CAD build for the part. Positions are in the model's coordinates, mm. A direction names the side the tool comes from. Give positions to 0.01 mm unless a question says otherwise; leave off trailing zeros. Order: outer loops, then holes, each group sorted by start corner. A loop starts at its lowest first (then second) coordinate and runs counter-clockwise, first axis right, second up. Notation, with made-up numbers: M 83.5,58 L 104.5,58 A29 cw 104.5,90 Z; hole C -8,-11.75 d4. An arc over 180 degrees is marked long. Put each result on its own line as item: value. Start each with the question number.
1) Cut at B-B (z = -1.5). Give the number of separate pieces and of enclosed holes in the cut face, and give its area (3 significant figures).
2) Pin check, flat tips, straight feed: pin 1 (5.5 mm diameter, centred on y = -20.5, z = -19, fed in from +X); pin 2 (9.5 mm diameter, centred on x = -62, y = -1.5, fed in from +Z); pin 3 (5.5 mm diameter, centred on x = 10.77, y = -29.6, fed in from -Z); pin 4 (4 mm diameter, centred on x = -26.57, y = 26.92, fed in from +Z). Stop position of each tip, or through.
3) Two-plate mould, pull along X, no slides. Class faces 1 (the face through (56.65, 5.06, -27.46)), 2 (the face through (-1, 1, 0)), 3 (the face through (50, 1, -15)): released by +X, released by -X, zero draft, split by the parting line, or undercut.
4) Drill centre lines: line 1 (X direction, y = -24.5, z = -27.5); line 2 (X direction, y = -0.5, z = -17.5); line 3 (Z direction, x = 61, y = 28.5). Where is each one in solid material? Low to high. Write a range as [from, to].
5) Cut at C-C (x = -40). Write the cut outline in (y, z), and give its area (3 significant figures).
6) Tool access for faces 4 (the face through (-56.65, 5.06, -27.46)), 5 (the face through (48.275, 0.672, -1.636)): list every direction of +Z, -Z, +X, -X, +Y, -Y with a clear straight run to the whole face (end or side of a thin tool).
7) Cut at A-A (z = -11). Write the cut outline in (x, y).
```python
from build123d import *

# Parameters (mm, degrees)
ESBO_O1_W                      = 100
ESBO_O1_H                      = 96
FLANGE_BASE1_DEPTH             = 5
ARESTA_FLANGE1_STRIP_W         = 21.4732
ARESTA_FLANGE1_STRIP_H         = 5
ARESTA_FLANGE1_STRIP_CUT_DEPTH = 96
ARESTA_FLANGE1_DEPTH           = 96
ARESTA_FLANGE2_STRIP_W         = 21.4732
ARESTA_FLANGE2_STRIP_H         = 5
ARESTA_FLANGE2_STRIP_CUT_DEPTH = 96
ARESTA_FLANGE2_DEPTH           = 96
ARESTA_FLANGE3_STRIP_W         = 21.4732
ARESTA_FLANGE3_STRIP_H         = 5
ARESTA_FLANGE3_STRIP_CUT_DEPTH = 96
ARESTA_FLANGE3_DEPTH           = 96
ARESTA_FLANGE4_STRIP_W         = 21.4732
ARESTA_FLANGE4_STRIP_H         = 5
ARESTA_FLANGE4_STRIP_CUT_DEPTH = 96
ARESTA_FLANGE4_DEPTH           = 96
FURO_DE_DI_METRO_4_2_4_2_1_D   = 4.2
PADR_OCIRCULAR1_COUNT          = 8
FURO_DE_DI_METRO_4_2_4_2_2_D   = 4.2
PADR_OCIRCULAR2_COUNT          = 8
FURO_DE_DI_METRO_4_2_4_2_3_D   = 4.2
PADR_OCIRCULAR3_COUNT          = 8
CORTE_EXTRUS_O1_REACH          = 90.482
PADR_O_LINEAR2_COUNT           = 6
PADR_O_LINEAR2_PITCH           = 15
ESPELHAR2_COPY_1_REACH         = 90.482
ESPELHAR2_COPY_2_REACH         = 90.482
ESPELHAR2_COPY_3_REACH         = 90.482
ESPELHAR2_COPY_4_REACH         = 90.482
ESPELHAR2_COPY_5_REACH         = 90.482


# Sheet-metal steps are written as plain solids
with BuildPart() as part:
    # Esboço1 → Flange-base1 (new body)
    with BuildSketch(Plane.XY):
        Rectangle(ESBO_O1_W, ESBO_O1_H)
    extrude(amount=-FLANGE_BASE1_DEPTH)

    # Aresta-Flange1 strip (across the edge) → Aresta-Flange1 strip cut (cut)
    with BuildSketch(Plane(origin=(50, 48, -5), x_dir=(-1, 0, 0), z_dir=(0, -1, 0))):
        with Locations((-5, -2.5)):
            Rectangle(ARESTA_FLANGE1_STRIP_W, ARESTA_FLANGE1_STRIP_H)
    extrude(amount=ARESTA_FLANGE1_STRIP_CUT_DEPTH, mode=Mode.SUBTRACT)

    # Aresta-Flange1 section (across the edge) → Aresta-Flange1 (add)
    with BuildSketch(Plane(origin=(50, 48, -5), x_dir=(-1, 0, 0), z_dir=(0, -1, 0))):
        with BuildLine():
            Line((0, 0.7366), (0, 25))
            Line((0, 25), (5, 25))
            Line((5, 25), (5, 0.7366))
            ThreePointArc((5, 0.7366), (5.215745145, 0.215745145), (5.7366, 0))
            Line((5.7366, 0), (5.7366, -5))
            ThreePointArc((5.7366, -5), (1.680211239, -3.319788761), (0, 0.7366))
        make_face()
    extrude(amount=ARESTA_FLANGE1_DEPTH)

    # Aresta-Flange2 strip (across the edge) → Aresta-Flange2 strip cut (cut)
    with BuildSketch(Plane(origin=(50, -48, -30), x_dir=(0, 0, 1), z_dir=(0, 1, 0))):
        with Locations((-5, -2.5)):
            Rectangle(ARESTA_FLANGE2_STRIP_W, ARESTA_FLANGE2_STRIP_H)
    extrude(amount=ARESTA_FLANGE2_STRIP_CUT_DEPTH, mode=Mode.SUBTRACT)

    # Aresta-Flange2 section (across the edge) → Aresta-Flange2 (add)
    with BuildSketch(Plane(origin=(50, -48, -30), x_dir=(0, 0, 1), z_dir=(0, 1, 0))):
        with BuildLine():
            Line((0, 0.7366), (0, 20))
            Line((0, 20), (5, 20))
            Line((5, 20), (5, 0.7366))
            ThreePointArc((5, 0.7366), (5.215745145, 0.215745145), (5.7366, 0))
            Line((5.7366, 0), (5.7366, -5))
            ThreePointArc((5.7366, -5), (1.680211239, -3.319788761), (0, 0.7366))
        make_face()
    extrude(amount=ARESTA_FLANGE2_DEPTH)

    # Aresta-Flange3 strip (across the edge) → Aresta-Flange3 strip cut (cut)
    with BuildSketch(Plane(origin=(-50, -48, -5), x_dir=(1, 0, 0), z_dir=(0, 1, 0))):
        with Locations((-5, -2.5)):
            Rectangle(ARESTA_FLANGE3_STRIP_W, ARESTA_FLANGE3_STRIP_H)
    extrude(amount=ARESTA_FLANGE3_STRIP_CUT_DEPTH, mode=Mode.SUBTRACT)

    # Aresta-Flange3 section (across the edge) → Aresta-Flange3 (add)
    with BuildSketch(Plane(origin=(-50, -48, -5), x_dir=(1, 0, 0), z_dir=(0, 1, 0))):
        with BuildLine():
            Line((0, 0.7366), (0, 25))
            Line((0, 25), (5, 25))
            Line((5, 25), (5, 0.7366))
            ThreePointArc((5, 0.7366), (5.215745145, 0.215745145), (5.7366, 0))
            Line((5.7366, 0), (5.7366, -5))
            ThreePointArc((5.7366, -5), (1.680211239, -3.319788761), (0, 0.7366))
        make_face()
    extrude(amount=ARESTA_FLANGE3_DEPTH)

    # Aresta-Flange4 strip (across the edge) → Aresta-Flange4 strip cut (cut)
    with BuildSketch(Plane(origin=(-50, 48, -30), x_dir=(0, 0, 1), z_dir=(0, -1, 0))):
        with Locations((-5, -2.5)):
            Rectangle(ARESTA_FLANGE4_STRIP_W, ARESTA_FLANGE4_STRIP_H)
    extrude(amount=ARESTA_FLANGE4_STRIP_CUT_DEPTH, mode=Mode.SUBTRACT)

    # Aresta-Flange4 section (across the edge) → Aresta-Flange4 (add)
    with BuildSketch(Plane(origin=(-50, 48, -30), x_dir=(0, 0, 1), z_dir=(0, -1, 0))):
        with BuildLine():
            Line((0, 0.7366), (0, 20))
            Line((0, 20), (5, 20))
            Line((5, 20), (5, 0.7366))
            ThreePointArc((5, 0.7366), (5.215745145, 0.215745145), (5.7366, 0))
            Line((5.7366, 0), (5.7366, -5))
            ThreePointArc((5.7366, -5), (1.680211239, -3.319788761), (0, 0.7366))
        make_face()
    extrude(amount=ARESTA_FLANGE4_DEPTH)

    # Furo de diâmetro Ø4.2 (4.2)1 (through all)
    with Locations(Plane(origin=(-10.773634515, 29.600317555, 0), x_dir=(1, 0, 0), z_dir=(0, 0, 1))):
        with Locations((0, 0)):
            furo_de_di_metro_4_2_4_2_1 = Hole(FURO_DE_DI_METRO_4_2_4_2_1_D / 2)

    # PadrãoCircular1: Furo de diâmetro Ø4.2 (4.2)1 ×8 about axis
    padr_ocircular1_axis = Axis((0, 0, 0), (0, 0, 1))
    for i in range(1, PADR_OCIRCULAR1_COUNT):
        add(furo_de_di_metro_4_2_4_2_1.rotate(padr_ocircular1_axis, i * 360 / PADR_OCIRCULAR1_COUNT), mode=Mode.SUBTRACT)

    # Furo de diâmetro Ø4.2 (4.2)2 (through all)
    with Locations(Plane(origin=(-6.817847839, 40.753324224, 0), x_dir=(1, 0, 0), z_dir=(0, 0, 1))):
        with Locations((0, 0)):
            furo_de_di_metro_4_2_4_2_2 = Hole(FURO_DE_DI_METRO_4_2_4_2_2_D / 2)

    # PadrãoCircular2: Furo de diâmetro Ø4.2 (4.2)2 ×8 about axis
    padr_ocircular2_axis = Axis((0, 10, 0), (0, 0, 1))
    for i in range(1, PADR_OCIRCULAR2_COUNT):
        add(furo_de_di_metro_4_2_4_2_2.rotate(padr_ocircular2_axis, i * 360 / PADR_OCIRCULAR2_COUNT), mode=Mode.SUBTRACT)

    # Furo de diâmetro Ø4.2 (4.2)3 (through all)
    with Locations(Plane(origin=(-6.817847839, 20.753324224, 0), x_dir=(1, 0, 0), z_dir=(0, 0, 1))):
        with Locations((0, 0)):
            furo_de_di_metro_4_2_4_2_3 = Hole(FURO_DE_DI_METRO_4_2_4_2_3_D / 2)

    # PadrãoCircular3: Furo de diâmetro Ø4.2 (4.2)3 ×8 about axis
    padr_ocircular3_axis = Axis((0, -10, 0), (0, 0, 1))
    for i in range(1, PADR_OCIRCULAR3_COUNT):
        add(furo_de_di_metro_4_2_4_2_3.rotate(padr_ocircular3_axis, i * 360 / PADR_OCIRCULAR3_COUNT), mode=Mode.SUBTRACT)

    # Esboço24 → Corte-extrusão1 (cut, up to next)
    with BuildSketch(Plane.XY.offset(-25), mode=Mode.PRIVATE) as corte_extrus_o1_sk1:
        with BuildLine():
            Line((-60.75, -37.4), (-59.25, -37.4))
            ThreePointArc((-59.25, -37.4), (-56.65, -40), (-59.25, -42.6))
            Line((-59.25, -42.6), (-60.75, -42.6))
            ThreePointArc((-60.75, -42.6), (-63.35, -40), (-60.75, -37.4))
        make_face()
    corte_extrus_o1_tool1 = extrude(corte_extrus_o1_sk1.sketch, amount=-CORTE_EXTRUS_O1_REACH, mode=Mode.PRIVATE) & part.part
    corte_extrus_o1 = corte_extrus_o1_tool1.solids().sort_by_distance((-60, -40, -25))[0]
    add(corte_extrus_o1, mode=Mode.SUBTRACT)

    # Padrão linear2: Corte-extrusão1 ×6
    with Locations(*[(0, i * PADR_O_LINEAR2_PITCH, 0) for i in range(1, PADR_O_LINEAR2_COUNT)]):
        add(corte_extrus_o1, mode=Mode.SUBTRACT)

    # Espelhar2: Corte-extrusão1 across plane
    add(corte_extrus_o1.mirror(Plane(origin=(0, 0, 0), x_dir=(0, 0, 1), z_dir=(1, 0, 0))), mode=Mode.SUBTRACT)

    # Espelhar2 copy 1 sketch → Espelhar2 copy 1 (cut, up to next)
    with BuildSketch(Plane(origin=(0, 15, -25), x_dir=(-1, 0, 0), z_dir=(0, 0, 1)), mode=Mode.PRIVATE) as espelhar2_copy_1_sk1:
        with BuildLine():
            Line((-60.75, 37.4), (-59.25, 37.4))
            ThreePointArc((-59.25, 37.4), (-56.65, 40), (-59.25, 42.6))
            Line((-59.25, 42.6), (-60.75, 42.6))
            ThreePointArc((-60.75, 42.6), (-63.35, 40), (-60.75, 37.4))
        make_face()
    espelhar2_copy_1_tool1 = extrude(espelhar2_copy_1_sk1.sketch, amount=-ESPELHAR2_COPY_1_REACH, mode=Mode.PRIVATE) & part.part
    add(espelhar2_copy_1_tool1.solids().sort_by_distance((60, -25, -25))[0], mode=Mode.SUBTRACT)

    # Espelhar2 copy 2 sketch → Espelhar2 copy 2 (cut, up to next)
    with BuildSketch(Plane(origin=(0, 30, -25), x_dir=(-1, 0, 0), z_dir=(0, 0, 1)), mode=Mode.PRIVATE) as espelhar2_copy_2_sk1:
        with BuildLine():
            Line((-60.75, 37.4), (-59.25, 37.4))
            ThreePointArc((-59.25, 37.4), (-56.65, 40), (-59.25, 42.6))
            Line((-59.25, 42.6), (-60.75, 42.6))
            ThreePointArc((-60.75, 42.6), (-63.35, 40), (-60.75, 37.4))
        make_face()
    espelhar2_copy_2_tool1 = extrude(espelhar2_copy_2_sk1.sketch, amount=-ESPELHAR2_COPY_2_REACH, mode=Mode.PRIVATE) & part.part
    add(espelhar2_copy_2_tool1.solids().sort_by_distance((60, -10, -25))[0], mode=Mode.SUBTRACT)

    # Espelhar2 copy 3 sketch → Espelhar2 copy 3 (cut, up to next)
    with BuildSketch(Plane(origin=(0, 45, -25), x_dir=(-1, 0, 0), z_dir=(0, 0, 1)), mode=Mode.PRIVATE) as espelhar2_copy_3_sk1:
        with BuildLine():
            Line((-60.75, 37.4), (-59.25, 37.4))
            ThreePointArc((-59.25, 37.4), (-56.65, 40), (-59.25, 42.6))
            Line((-59.25, 42.6), (-60.75, 42.6))
            ThreePointArc((-60.75, 42.6), (-63.35, 40), (-60.75, 37.4))
        make_face()
    espelhar2_copy_3_tool1 = extrude(espelhar2_copy_3_sk1.sketch, amount=-ESPELHAR2_COPY_3_REACH, mode=Mode.PRIVATE) & part.part
    add(espelhar2_copy_3_tool1.solids().sort_by_distance((60, 5, -25))[0], mode=Mode.SUBTRACT)

    # Espelhar2 copy 4 sketch → Espelhar2 copy 4 (cut, up to next)
    with BuildSketch(Plane(origin=(0, 60, -25), x_dir=(-1, 0, 0), z_dir=(0, 0, 1)), mode=Mode.PRIVATE) as espelhar2_copy_4_sk1:
        with BuildLine():
            Line((-60.75, 37.4), (-59.25, 37.4))
            ThreePointArc((-59.25, 37.4), (-56.65, 40), (-59.25, 42.6))
            Line((-59.25, 42.6), (-60.75, 42.6))
            ThreePointArc((-60.75, 42.6), (-63.35, 40), (-60.75, 37.4))
        make_face()
    espelhar2_copy_4_tool1 = extrude(espelhar2_copy_4_sk1.sketch, amount=-ESPELHAR2_COPY_4_REACH, mode=Mode.PRIVATE) & part.part
    add(espelhar2_copy_4_tool1.solids().sort_by_distance((60, 20, -25))[0], mode=Mode.SUBTRACT)

    # Espelhar2 copy 5 sketch → Espelhar2 copy 5 (cut, up to next)
    with BuildSketch(Plane(origin=(0, 75, -25), x_dir=(-1, 0, 0), z_dir=(0, 0, 1)), mode=Mode.PRIVATE) as espelhar2_copy_5_sk1:
        with BuildLine():
            Line((-60.75, 37.4), (-59.25, 37.4))
            ThreePointArc((-59.25, 37.4), (-56.65, 40), (-59.25, 42.6))
            Line((-59.25, 42.6), (-60.75, 42.6))
            ThreePointArc((-60.75, 42.6), (-63.35, 40), (-60.75, 37.4))
        make_face()
    espelhar2_copy_5_tool1 = extrude(espelhar2_copy_5_sk1.sketch, amount=-ESPELHAR2_COPY_5_REACH, mode=Mode.PRIVATE) & part.part
    add(espelhar2_copy_5_tool1.solids().sort_by_distance((60, 35, -25))[0], mode=Mode.SUBTRACT)


solid = part.part
```
Solution:
1. separate pieces: 1
1. enclosed holes: 24
1. area: 8,910 mm²
2. pin 1: x = 50
2. pin 2: z = -25
2. pin 3: z = -5
2. pin 4: through
3. face 1: undercut
3. face 2: zero draft
3. face 3: released by +X
4. line 1: [-70, -63.3], [-56.7, -46], [46, 56.7], [63.3, 70]
4. line 2: [-50, -45], [45, 50]
4. line 3: [-30, -25]
5. outline: M -48,-5 L 48,-5 L 48,0 L -48,0 Z
5. area: 480 mm²
6. face 4: +Z, -Z
6. face 5: +Z, +X, +Y, -Y
7. outline: M -50,-48 L -45,-48 L -45,48 L -50,48 Z; M 45,-48 L 50,-48 L 50,48 L 45,48 Z
